The model under review builds one solid part; all positions refer to its coordinate system, in mm. A direction names the side the tool comes from. Coordinates: 2 decimals unless noted, no trailing zeros. Loops run counter-clockwise (first coordinate to the right, second up) from the corner with the lowest first, then second, coordinate; pieces in that order, holes last. Notation, with made-up numbers: M 86.25,64 L 113.25,64 A15 ccw 113.25,93 Z; hole C 20,4.25 d6. An arc over 180 degrees is marked long. Use one line per item in the form item = value.
```python
from build123d import *

# Parameters (mm, degrees)
CROQUIS1_R              = 10.5
CROQUIS1_R_2            = 1.5
SALIENTE_EXTRUIR1_DEPTH = 2.5
CROQUIS2_R              = 4
CROQUIS2_R_2            = 3
SALIENTE_EXTRUIR2_DEPTH = 3.5
CROQUIS3_R              = 0.75
CORTAR_EXTRUIR1_DEPTH   = 3.5


with BuildPart() as part:
    # Croquis1 → Saliente-Extruir1 (new body)
    with BuildSketch(Plane.XY):
        Circle(CROQUIS1_R)
        Circle(CROQUIS1_R_2, mode=Mode.SUBTRACT)
    extrude(amount=SALIENTE_EXTRUIR1_DEPTH)

    # Croquis2 → Saliente-Extruir2 (add)
    with BuildSketch(Plane.XY.offset(2.5)):
        Circle(CROQUIS2_R)
        Circle(CROQUIS2_R_2, mode=Mode.SUBTRACT)
    extrude(amount=SALIENTE_EXTRUIR2_DEPTH)

    # Croquis3 → Cortar-Extruir1 (cut)
    with BuildSketch(Plane.XY.offset(2.5)):
        with Locations((-7.75, 0)):
            Circle(CROQUIS3_R)
        with Locations((-7.75, 3.5)):
            Circle(CROQUIS3_R)
        with Locations((-7.75, -3.5)):
            Circle(CROQUIS3_R)
        with Locations((3.5, 7.75)):
            Circle(CROQUIS3_R)
        with Locations((0, 7.75)):
            Circle(CROQUIS3_R)
        with Locations((-3.5, 7.75)):
            Circle(CROQUIS3_R)
        with Locations((7.75, -3.5)):
            Circle(CROQUIS3_R)
        with Locations((7.75, 0)):
            Circle(CROQUIS3_R)
        with Locations((7.75, 3.5)):
            Circle(CROQUIS3_R)
        with Locations((-3.5, -7.75)):
            Circle(CROQUIS3_R)
        with Locations((0, -7.75)):
            Circle(CROQUIS3_R)
        with Locations((3.5, -7.75)):
            Circle(CROQUIS3_R)
    extrude(amount=-CORTAR_EXTRUIR1_DEPTH, mode=Mode.SUBTRACT)


solid = part.part
```
1. The part is to be moulded in two halves that separate along X. For faces 1 (the face through (10, 3.2, 1.2)), 2 (the face through (1, 3, 6)), 3 (the face through (-8.5, -3.5, 1.3)), say which applies: pulls with the +X half, pulls with the -X half, needs draft (parallel to the pull), parting line crosses it, or undercut.
Response values:
face_1 = parting line crosses it
face_2 = needs draft
face_3 = undercut
2. Insertion check: P1, Ø1.4, axis at x = -3.5, y = -7.75, coming from the -Z side; P2, Ø1.7, axis at x = -7.75, y = -3.5, coming from the +Z side; P3, Ø3, axis at y = 2, z = 4.5, coming from the +X side; P4, Ø1.5, axis at y = 6.5, z = 1.5, coming from the +X side. Each pin has a flat end and moves straight along its axis. Give the tip position at first contact, or say it passes through.
Response values:
P1 = through
P2 = 2.5
P3 = 3.97
P4 = 8.79
3. Wall thickness on line 1 along Y through (x, z) = (0.5, 1.7); line 2 along Y through (x, z) = (-7.75, 1.35); line 3 along X through (y, z) = (0.25, 2.25): over which ranges is each line inside the solid? List them lowest first. Write a range as from..to.
Response values:
line_1 = -10.49..-8.31, -7.19..-1.41, 1.41..7.19, 8.31..10.49
line_2 = -7.08..-4.25, -2.75..-0.75, 0.75..2.75, 4.25..7.08
line_3 = -10.5..-8.46, -7.04..-1.48, 1.48..7.04, 8.46..10.5
4. Add section D-D (x = 3.5). State the section outline as (y, z) points, then the cut area to 3 significant figures.
Response values:
outline = M -9.9,0 L -8.5,0 L -8.5,2.5 L -9.9,2.5 Z; M -7,0 L 7,0 L 7,2.5 L 1.94,2.5 L 1.94,6 L -1.94,6 L -1.94,2.5 L -7,2.5 Z; M 8.5,0 L 9.9,0 L 9.9,2.5 L 8.5,2.5 Z
area = 55.6 mm^2
5. Add section A-A (y = 0). State the section outline as (x, z) points.
Response values:
outline = M -10.5,0 L -8.5,0 L -8.5,2.5 L -10.5,2.5 Z; M -7,0 L -1.5,0 L -1.5,2.5 L -3,2.5 L -3,6 L -4,6 L -4,2.5 L -7,2.5 Z; M 1.5,0 L 7,0 L 7,2.5 L 4,2.5 L 4,6 L 3,6 L 3,2.5 L 1.5,2.5 Z; M 8.5,0 L 10.5,0 L 10.5,2.5 L 8.5,2.5 Z
6. Machinability: for faces 4 (the face through (1.3, -1.3, 2.5)), 5 (the face through (7.155, -3.956, 1.268)), which of the approach directions +Z, -Z, +X, -X, +Y, -Y give a long, thin tool a straight path to every point of the face, cutting with its end or side? Answer none if there is none.
Response values:
face_4 = +Z
face_5 = +Z, -Z
7. Add section C-C (z = 0.4). Count the separate pieces of the cut face and the enclosed holes in it, then the cut area to 3 significant figures.
Response values:
separate_pieces = 1
enclosed_holes = 13
area = 318 mm^2
